from build123d import *

# Parameters (mm, degrees)
SKETCH1_W             = 248.25
SKETCH1_H             = 19.05
BOSS_EXTRUDE1_DEPTH   = 38.1
HOLE1_D               = 3.175
HOLE1_DEPTH           = 31.75
HOLE1_CSINK_D         = 10.16
HOLE1_CSINK_ANGLE     = 82
HOLE1_TIP             = 0.953866233
HOLE2_D               = 3.175
HOLE2_DEPTH           = 57.15
HOLE2_CSINK_D         = 10.16
HOLE2_CSINK_ANGLE     = 82
HOLE2_TIP             = 0.953866233
SKETCH6_W             = 248.25
SKETCH6_H             = 20.637862114
BOSS_EXTRUDE3_DEPTH   = 19.05
F_8_CLEARANCE_HOLE1_D = 4.9149


with BuildPart() as part:
    # Sketch1 → Boss-Extrude1 (new body)
    with BuildSketch(Plane.XY):
        with Locations((124.125, 47.625)):
            Rectangle(SKETCH1_W, SKETCH1_H)
    extrude(amount=BOSS_EXTRUDE1_DEPTH)

    # Hole1
    with Locations(Plane(origin=(-1090.512770337, -52.974999997, -12.7), x_dir=(0, 1, 0), z_dir=(0, 0, -1))):
        with Locations((-100.332047386, 1313.362770337), (100.599999997, 1313.362770337), (100.599999997, 1115.912770337), (100.599999997, 1214.637770337), (-100.332047386, 1214.637770337), (-100.332047386, 1115.912770337)):
            CounterSinkHole(HOLE1_D / 2, HOLE1_CSINK_D / 2, depth=HOLE1_DEPTH, counter_sink_angle=HOLE1_CSINK_ANGLE)
            with Locations((0, 0, -(HOLE1_DEPTH + HOLE1_TIP / 2))):  # 118° drill point
                Cone(0, HOLE1_D / 2, HOLE1_TIP, mode=Mode.SUBTRACT)

    # Hole2
    with Locations(Plane(origin=(-1090.512770337, 57.15, -415.792401694), x_dir=(0.3746065934159092, 0, 0.9271838545667885), z_dir=(0, 1, 0))):
        with Locations((848.944412528, 940.413642522), (885.927448463, 1031.949868564), (867.435930496, 986.181755543), (830.452894561, 894.645529501)):
            CounterSinkHole(HOLE2_D / 2, HOLE2_CSINK_D / 2, depth=HOLE2_DEPTH, counter_sink_angle=HOLE2_CSINK_ANGLE)
            with Locations((0, 0, -(HOLE2_DEPTH + HOLE2_TIP / 2))):  # 118° drill point
                Cone(0, HOLE2_D / 2, HOLE2_TIP, mode=Mode.SUBTRACT)

    # Sketch6 → Boss-Extrude3 (add)
    with BuildSketch(Plane(origin=(0, 57.15, 0), x_dir=(1, 0, 0), z_dir=(0, 1, 0))):
        with Locations((124.125, -48.418931057)):
            Rectangle(SKETCH6_W, SKETCH6_H)
    extrude(amount=-BOSS_EXTRUDE3_DEPTH)

    # #8 Clearance Hole1 (through all)
    with Locations(Plane(origin=(0, 57.15, 0), x_dir=(1, 0, 0), z_dir=(0, 1, 0))):
        with Locations((12.7, -46.037862114), (203.2, -46.037862114)):
            Hole(F_8_CLEARANCE_HOLE1_D / 2)


solid = part.part
Verification items for the finished model (mm, model axes). Give positions to 0.01 mm unless a question says otherwise; leave off trailing zeros.
1) Thickness scan on line 1 along X through (y, z) = (44.5, 19.05); line 2 along Z through (x, y) = (12.7, 42.5); line 3 along X through (y, z) = (48.75, 19.5). Record the ranges inside material, lowest first.
2) Draft check along Z on faces 1 (the flat face through (122, 38.1, 29)), 2 (the conical face through (196.42, 53.33, 18.88)), 3 (the flat face through (122, 48, 58.738)), 4 (the conical face through (51.67, 53.33, 19.81)). Enter one of: pulls with the +Z half, pulls with the -Z half, needs draft (parallel to the pull), parting line crosses it, or undercut.
3) Depth check by flat-ended pin: pin 1 Ø3.5 at (x, z) = (99.44, 19.05) entering from +Y; pin 2 Ø4 at (x, z) = (198.17, 19.05) entering from +Y; pin 3 Ø1.9 at (x, y) = (25.4, 47.625) entering from -Z. Enter the tip coordinate at first touch or a pass-through.
Answers:
1. line 1: x = 0 to 48.49, 51.67 to 97.86, 101.03 to 147.22, 150.39 to 196.58, 199.76 to 248.25
1. line 2: z = 0 to 43.58, 48.5 to 58.74
1. line 3: x = 0 to 48.56, 51.6 to 97.92, 100.97 to 147.28, 150.33 to 196.65, 199.69 to 248.25
2. face 1: needs draft
2. face 2: undercut
2. face 3: pulls with the +Z half
2. face 4: undercut
3. pin 1: stops at y = 53.32
3. pin 2: stops at y = 53.61
3. pin 3: stops at z = 19.43
